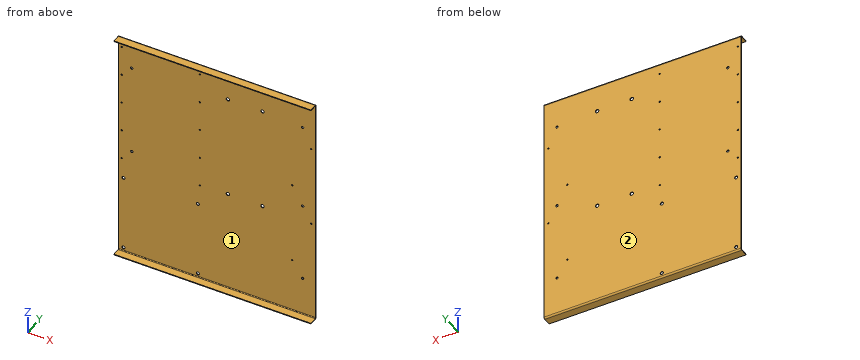
```python
from build123d import *

# Parameters (mm, degrees)
SKETCH_1_W                         = 285
SKETCH_1_H                         = 337
SM_BASE_FLANGE_1_DEPTH             = 1
SM_EDGE_FLANGE_1_STRIP_W           = 6.2
SM_EDGE_FLANGE_1_STRIP_H           = 1
SM_EDGE_FLANGE_1_STRIP_CUT_DEPTH   = 285
SM_EDGE_FLANGE_1_STRIP_2_W         = 6.2
SM_EDGE_FLANGE_1_STRIP_2_H         = 1
SM_EDGE_FLANGE_1_STRIP_CUT_2_DEPTH = 285
SM_EDGE_FLANGE_1_DEPTH             = 285
SM_EDGE_FLANGE_1_BEND_DEPTH        = 285
SKETCH_10_R                        = 1
CUT_EXTRUDE_1_DEPTH                = 10
SKETCH_11_R                        = 2.25
CUT_EXTRUDE_2_DEPTH                = 3
SKETCH_12_R                        = 1.75
CUT_EXTRUDE_3_DEPTH                = 3
SKETCH_13_R                        = 2.5
CUT_EXTRUDE_4_DEPTH                = 10


# Sheet-metal steps are written as plain solids
with BuildPart() as part:
    # Sketch 1 → Базовая кромка1 (new body)
    with BuildSketch(Plane(origin=(0, 0, 0), x_dir=(1, 0, 0), z_dir=(0, 1, 0))):
        with Locations((110.522140356, -133.470311428)):
            Rectangle(SKETCH_1_W, SKETCH_1_H)
    extrude(amount=-SM_BASE_FLANGE_1_DEPTH)

    # Ребро-кромка1 strip (across the edge) → Ребро-кромка1 strip cut (cut)
    with BuildSketch(Plane(origin=(253.022140356, -1, 301.970311428), x_dir=(0, 0, -1), z_dir=(-1, 0, 0))):
        with Locations((-2, -0.5)):
            Rectangle(SM_EDGE_FLANGE_1_STRIP_W, SM_EDGE_FLANGE_1_STRIP_H)
    extrude(amount=SM_EDGE_FLANGE_1_STRIP_CUT_DEPTH, mode=Mode.SUBTRACT)

    # Ребро-кромка1 strip 2 (across the edge) → Ребро-кромка1 strip cut 2 (cut)
    with BuildSketch(Plane(origin=(-31.977859644, -1, -35.029688572), x_dir=(0, 0, 1), z_dir=(1, 0, 0))):
        with Locations((-2, -0.5)):
            Rectangle(SM_EDGE_FLANGE_1_STRIP_2_W, SM_EDGE_FLANGE_1_STRIP_2_H)
    extrude(amount=SM_EDGE_FLANGE_1_STRIP_CUT_2_DEPTH, mode=Mode.SUBTRACT)

    # Ребро-кромка1 section (across the edge) → Ребро-кромка1 (add)
    with BuildSketch(Plane(origin=(253.022140356, -1, 301.970311428), x_dir=(0, 0, -1), z_dir=(-1, 0, 0))):
        with BuildLine():
            Line((-1, 1.1), (-1, 12))
            Line((-1, 12), (0, 12))
            Line((0, 12), (0, 1.1))
            ThreePointArc((0, 1.1), (0.322182541, 0.322182541), (1.1, 0))
            Line((1.1, 0), (1.1, -1))
            ThreePointArc((1.1, -1), (-0.38492424, -0.38492424), (-1, 1.1))
        make_face()
    extrude(amount=SM_EDGE_FLANGE_1_DEPTH)

    # Ребро-кромка1 section 2 (across the edge) → Ребро-кромка1 bend (add)
    with BuildSketch(Plane(origin=(-31.977859644, -1, -35.029688572), x_dir=(0, 0, 1), z_dir=(1, 0, 0))):
        with BuildLine():
            Line((-1, 1.1), (-1, 12))
            Line((-1, 12), (0, 12))
            Line((0, 12), (0, 1.1))
            ThreePointArc((0, 1.1), (0.322182541, 0.322182541), (1.1, 0))
            Line((1.1, 0), (1.1, -1))
            ThreePointArc((1.1, -1), (-0.38492424, -0.38492424), (-1, 1.1))
        make_face()
    extrude(amount=SM_EDGE_FLANGE_1_BEND_DEPTH)

    # Эскиз10 → Вырез-Вытянуть1 (cut)
    with BuildSketch(Plane(origin=(0, 0, 0), x_dir=(1, 0, 0), z_dir=(0, 1, 0))):
        with Locations(Location((-27.477859644, -110.970311428, 0), (0, 0, 270))):
            Circle(SKETCH_10_R)
        with Locations(Location((85.522140356, -110.970311428, 0), (0, 0, 270))):
            Circle(SKETCH_10_R)
        with Locations(Location((85.522140356, -154.970311428, 0), (0, 0, 270))):
            Circle(SKETCH_10_R)
        with Locations(Location((-27.477859644, -154.970311428, 0), (0, 0, 270))):
            Circle(SKETCH_10_R)
        with Locations(Location((-27.477859644, -198.970311428, 0), (0, 0, 270))):
            Circle(SKETCH_10_R)
        with Locations(Location((85.522140356, -198.970311428, 0), (0, 0, 270))):
            Circle(SKETCH_10_R)
        with Locations(Location((-27.477859644, -242.970311428, 0), (0, 0, 270))):
            Circle(SKETCH_10_R)
        with Locations(Location((85.522140356, -242.970311428, 0), (0, 0, 270))):
            Circle(SKETCH_10_R)
        with Locations(Location((85.522140356, -286.970311428, 0), (0, 0, 270))):
            Circle(SKETCH_10_R)
        with Locations(Location((-27.477859644, -286.970311428, 0), (0, 0, 270))):
            Circle(SKETCH_10_R)
        with Locations(Location((246.522140356, -230.720311428, 0), (0, 0, 270))):
            Circle(SKETCH_10_R)
        with Locations(Location((219.022140356, -162.720311428, 0), (0, 0, 270))):
            Circle(SKETCH_10_R)
        with Locations(Location((246.522140356, -112.220311428, 0), (0, 0, 270))):
            Circle(SKETCH_10_R)
        with Locations(Location((219.022140356, -44.220311428, 0), (0, 0, 270))):
            Circle(SKETCH_10_R)
    extrude(amount=-CUT_EXTRUDE_1_DEPTH, mode=Mode.SUBTRACT)

    # Эскиз11 → Вырез-Вытянуть2 (cut)
    with BuildSketch(Plane(origin=(0, 0, 0), x_dir=(1, 0, 0), z_dir=(0, 1, 0))):
        with Locations(Location((82.522140356, 29.529688572, 0), (0, 0, 270))):
            Circle(SKETCH_11_R)
        with Locations(Location((82.522140356, -80.470311428, 0), (0, 0, 270))):
            Circle(SKETCH_11_R)
        with Locations(Location((-24.977859644, -80.470311428, 0), (0, 0, 270))):
            Circle(SKETCH_11_R)
        with Locations(Location((-24.977859644, 29.529688572, 0), (0, 0, 270))):
            Circle(SKETCH_11_R)
    extrude(amount=-CUT_EXTRUDE_2_DEPTH, mode=Mode.SUBTRACT)

    # Эскиз12 → Вырез-Вытянуть3 (cut)
    with BuildSketch(Plane(origin=(0, 0, 0), x_dir=(1, 0, 0), z_dir=(0, 1, 0))):
        with Locations(Location((-12.977859644, -126.970311428, 0), (0, 0, 270))):
            Circle(SKETCH_12_R)
        with Locations(Location((234.022140356, -20.970311428, 0), (0, 0, 270))):
            Circle(SKETCH_12_R)
        with Locations(Location((234.022140356, -135.470311428, 0), (0, 0, 270))):
            Circle(SKETCH_12_R)
        with Locations(Location((-12.977859644, -258.970311428, 0), (0, 0, 270))):
            Circle(SKETCH_12_R)
        with Locations(Location((234.022140356, -259.970311428, 0), (0, 0, 270))):
            Circle(SKETCH_12_R)
    extrude(amount=-CUT_EXTRUDE_3_DEPTH, mode=Mode.SUBTRACT)

    # Эскиз13 → Вырез-Вытянуть4 (cut)
    with BuildSketch(Plane.XZ.offset(1)):
        with Locations(Location((126.022140356, 262.970311428, 0), (0, 0, 270))):
            Circle(SKETCH_13_R)
        with Locations(Location((176.022140356, 262.970311428, 0), (0, 0, 270))):
            Circle(SKETCH_13_R)
        with Locations(Location((126.022140356, 112.970311428, 0), (0, 0, 270))):
            Circle(SKETCH_13_R)
        with Locations(Location((176.022140356, 112.970311428, 0), (0, 0, 270))):
            Circle(SKETCH_13_R)
    extrude(amount=-CUT_EXTRUDE_4_DEPTH, mode=Mode.SUBTRACT)


solid = part.part
```
Work out the finished part from the listing and answer in its coordinate system (mm). Face numbers are marked on the shaded views. A direction names the side the tool comes from. Round coordinates to 2 decimals unless told otherwise and drop trailing zeros. Loops run counter-clockwise (first coordinate to the right, second up) from the corner with the lowest first, then second, coordinate; pieces in that order, holes last.
(1) The part is cut by section B-B, the plane x = -7. Give the vertices of the cut face in (y, z), and give its area (3 significant figures).
Computed values:
outline: (-13, -36.03) - (-2.1, -36.03) arc R2.1 ccw to (0, -33.93) - (0, 300.87) arc R2.1 ccw to (-2.1, 302.97) - (-13, 302.97) - (-13, 301.97) - (-2.1, 301.97) arc R1.1 cw to (-1, 300.87) - (-1, -33.93) arc R1.1 cw to (-2.1, -35.03) - (-13, -35.03) - close
area: 362 mm2
(2) Find the intervals of material crossed by L1, parallel to Z at x = 32, y = -10; L2, parallel to Y at x = 83, z = 249; L3, parallel to Z at x = 116.5, y = -1.25, in increasing order.
Computed values:
L1: z = -36.03 to -35.03, 301.97 to 302.97
L2: y = -1 to 0
L3: z = -35.85 to -34.63, 301.57 to 302.79
(3) This flat-tipped pin is pushed along its axis until it touches: P1, Ø1, axis at x = 146.5, z = 225, coming from the -Y side. Where does it stop, or does it pass through?
Computed values:
P1: stops at y = -1
(4) The part is cut by section C-C, the plane z = 209. Give the vertices of the cut face in (x, y), and give its area (3 significant figures).
Computed values:
outline: (-31.98, -1) - (253.02, -1) - (253.02, 0) - (-31.98, 0) - close
area: 285 mm2
(5) For the marked faces 1 and 2, determine the directions among +Z, -Z, +X, -X, +Y, -Y from which every point of the face is accessible in a straight line to the end or side of a thin tool.
Computed values:
face 1: +X, -X, -Y
face 2: +Z, -Z, +X, -X, +Y
(6) The part is cut by section A-A, the plane y = -4.5. Give the vertices of the cut face in (x, z), and give its area (3 significant figures).
Computed values:
outline: (-31.98, -36.03) - (253.02, -36.03) - (253.02, -35.03) - (-31.98, -35.03) - close; (-31.98, 301.97) - (253.02, 301.97) - (253.02, 302.97) - (-31.98, 302.97) - close
area: 570 mm2
